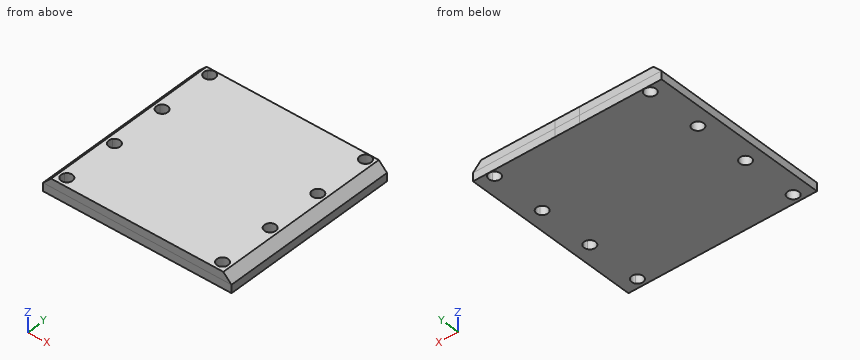
Autodesk Inventor part; units mm, degrees
ref_plane "YZ Plane" through (0, 0, 0) normal (1, 0, 0) x (0, 1, 0)
ref_plane "XZ Plane" through (0, 0, 0) normal (0, 1, 0) x (-1, 0, 0)
ref_plane "XY Plane" through (0, 0, 0) normal (0, 0, 1) x (1, 0, 0)
sketch "Sketch1" plane through (0, 0, 0) normal (0, 0, 1) x (1, 0, 0)
  line L0 (0, 0) -> (15, 0)
  arc A0 (-42.9289, -5.4718) -> (-42.9289, -1.7934) centre (-40, -3.6326) ccw
  arc A1 (-42.9289, -38.9718) -> (-42.9289, -35.2934) centre (-40, -37.1326) ccw
  arc A2 (-42.9289, -72.4718) -> (-42.9289, -68.7934) centre (-40, -70.6326) ccw
  arc A3 (-42.9289, -105.9718) -> (-42.9289, -102.2934) centre (-40, -104.1326) ccw
  arc A4 (57.9289, -102.2934) -> (57.9289, -105.9718) centre (55, -104.1326) ccw
  arc A5 (57.9289, -68.7934) -> (57.9289, -72.4718) centre (55, -70.6326) ccw
  arc A6 (57.9289, -35.2934) -> (57.9289, -38.9718) centre (55, -37.1326) ccw
  arc A7 (57.9289, -1.7934) -> (57.9289, -5.4718) centre (55, -3.6326) ccw
  line L1 (0, 0) -> (15, 0)
  spline S0 degree 3 poles (-42.9289, -5.4718) (-43.0252, -5.3184) (-43.1102, -5.1562) (-43.3669, -4.5537) (-43.4585, -4.079) (-43.4585, -3.1862) (-43.3669, -2.7114) (-43.1102, -2.109) (-43.0252, -1.9468) (-42.9289, -1.7934) knots 1.816211 1.816211 1.816211 1.816211 1.867954 1.867954 2.001868 2.001868 2.135782 2.135782 2.187525 2.187525 2.187525 2.187525
  spline S1 degree 3 poles (-42.9289, -105.9718) (-43.0252, -105.8184) (-43.1102, -105.6562) (-43.3669, -105.0537) (-43.4585, -104.579) (-43.4585, -103.6862) (-43.3669, -103.2114) (-43.1102, -102.609) (-43.0252, -102.4468) (-42.9289, -102.2934) knots 1.816211 1.816211 1.816211 1.816211 1.867954 1.867954 2.001868 2.001868 2.135782 2.135782 2.187525 2.187525 2.187525 2.187525
  spline S2 degree 3 poles (-42.9289, -72.4718) (-43.0252, -72.3184) (-43.1102, -72.1562) (-43.3669, -71.5537) (-43.4585, -71.079) (-43.4585, -70.1862) (-43.3669, -69.7114) (-43.1102, -69.109) (-43.0252, -68.9468) (-42.9289, -68.7934) knots 1.816211 1.816211 1.816211 1.816211 1.867954 1.867954 2.001868 2.001868 2.135782 2.135782 2.187525 2.187525 2.187525 2.187525
  spline S3 degree 3 poles (-42.9289, -38.9718) (-43.0252, -38.8184) (-43.1102, -38.6562) (-43.3669, -38.0537) (-43.4585, -37.579) (-43.4585, -36.6862) (-43.3669, -36.2114) (-43.1102, -35.609) (-43.0252, -35.4468) (-42.9289, -35.2934) knots 1.816211 1.816211 1.816211 1.816211 1.867954 1.867954 2.001868 2.001868 2.135782 2.135782 2.187525 2.187525 2.187525 2.187525
  arc A8 (57.9289, -38.9718) -> (57.9289, -35.2934) centre (55, -37.1326) ccw
  arc A9 (57.9289, -5.4718) -> (57.9289, -1.7934) centre (55, -3.6326) ccw
  arc A10 (57.9289, -72.4718) -> (57.9289, -68.7934) centre (55, -70.6326) ccw
  arc A11 (57.9289, -105.9718) -> (57.9289, -102.2934) centre (55, -104.1326) ccw
  line L2 (-50, 0.0004) -> (65, 0.0004)
  line L3 (65, 0.0004) -> (65, -109.3496)
  line L4 (65, -109.3496) -> (-50, -109.3496)
  line L5 (-50, -109.3496) -> (-50, 0.0004)
  point P0 (7.5, -111.1326)
  point P1 (84.0033, -110.1193)
  point P2 (84.0033, -111.5873)
  point P3 (-42.9289, -102.2934)
  point P4 (84.0033, -151.6974)
  point P5 (84.0033, -136.8593)
  point P6 (84.0033, -138.3274)
  point P7 (84.0033, -123.4893)
  point P8 (84.0033, -124.9573)
  point P9 (7.5, -109.3496)
  point P10 (-42.9289, -35.2934)
  dimension "d8" = 115
  dimension "d9" = 109.35
  dimension "d10" = 3.633
extrude "Extrusion1" add sketch "Sketch1" along normal mid plane 10
chamfer "Chamfer1" distance 5 angle 45 2 edges at (-50, -54.6746, 5) (65, -54.6746, 5)
properties part number "Upper cover of robot head" material "Steel, Alloy"
Build history of the part. All positions in model axes, mm. Round coordinates to 2 decimals unless told otherwise and drop trailing zeros. Write each loop counter-clockwise with the first axis right and the second up, starting at its lowest first coordinate (ties: lowest second). Pieces come first, ordered by that corner, then holes. Notation, with made-up numbers: M -28.75,-23.5 L -13.75,-23.5 A32 cw -13.75,9.5 Z; hole C 8,-20 d6. An arc over 180 degrees is marked long. Answer as a JSON object with one key per item and string values. Group by question number.
(1) Drill centre lines: L1, parallel to Y at x = -40, z = 1.8; L2, parallel to Y at x = 56.5, z = 1.5; L3, parallel to X at y = -27, z = 0.25. Where is each one in solid material? Low to high.
(2) Cut at B-B (z = -2). Give the number of separate pieces and of enclosed holes in the cut face, and give its area (3 significant figures).
(3) Flat gauge pin, fed straight in: pin 1 (3 mm diameter, centred on y = -83, z = 4, fed in from +X). Where does the tip first touch, or does it go through?
(4) Cut at A-A (x = -40). Give the cut face in (y, z).
(5) Cut at C-C (x = 55.5). Give the cut face in (y, z).
Responses:
{
 "1": {"L1": "y = -109.35 to -107.59, -100.67 to -74.09, -67.17 to -40.59, -33.67 to -7.09, -0.17 to 0", "L2": "y = -109.35 to -107.25, -101.02 to -73.75, -67.52 to -40.25, -34.02 to -6.75, -0.52 to 0", "L3": "x = -49.75 to 64.75"},
 "2": {"separate pieces": "1", "enclosed holes": "8", "area": "12,300 mm2"},
 "3": {"pin 1": "stops at x = 62.5"},
 "4": {"outline": "M -109.35,-5 L -107.59,-5 L -107.59,5 L -109.35,5 Z; M -100.67,-5 L -74.09,-5 L -74.09,5 L -100.67,5 Z; M -67.17,-5 L -40.59,-5 L -40.59,5 L -67.17,5 Z; M -33.67,-5 L -7.09,-5 L -7.09,5 L -33.67,5 Z; M -0.17,-5 L 0,-5 L 0,5 L -0.17,5 Z"},
 "5": {"outline": "M -109.35,-5 L -107.55,-5 L -107.55,5 L -109.35,5 Z; M -100.71,-5 L -74.05,-5 L -74.05,5 L -100.71,5 Z; M -67.21,-5 L -40.55,-5 L -40.55,5 L -67.21,5 Z; M -33.71,-5 L -7.05,-5 L -7.05,5 L -33.71,5 Z; M -0.21,-5 L 0,-5 L 0,5 L -0.21,5 Z"}
}
